Check sheet for the modelled part. Datum: model origin and axes. Units: mm. A direction names the side the tool comes from. Give positions to 0.01 mm unless a question says otherwise; leave off trailing zeros. Loops run counter-clockwise (first coordinate to the right, second up) from the corner with the lowest first, then second, coordinate; pieces in that order, holes last. Notation, with made-up numbers: (-8, 70) -> (8, 70) arc R22 ccw to (8, 94) -> close; hole circle Ø5 at (71, -21.75). An arc over 180 degrees is marked (long way). Answer as CSV lines item,"result". Start each with the question number.
(1) Release check for a two-part mould opening along X. For faces 1 (the face through (3, 6.588, 0)), 2 (the face through (0, 5.588, 0)), 3 (the face through (-0.24, -17.844, 0.462)) record: pulls with the +X half, pulls with the -X half, needs draft (parallel to the pull), parting line crosses it, or undercut.
(2) Gauge pin test, flat ends, axial feed: pin 1 Ø3 at (x, y) = (2, -9) entering from +Z; pin 2 Ø1.5 at (x, y) = (-3, -10.5) entering from +Z; pin 3 Ø2 at (y, z) = (2, 0) entering from +X. Record the tip position at first contact, or that the pin passes through.
(3) Section check A-A on y = -8.75. Enter the section's corners in (x, z), plus the area to 3 significant figures.
(4) Material ranges on line 1 (Z direction, x = 0, y = -6); line 2 (Y direction, x = 5.75, z = -0.75); line 3 (Y direction, x = 0, z = -4.75), recorded low to high. Write a range as from..to.
(5) Access from +Z, -Z, +X, -X, +Y, -Y to the whole of each face (thin tool, end or side, straight path). Record for faces 4 (the face through (-2.86, -7.29, -0.9)), 5 (the face through (-3, 6.588, 0)), 6 (the face through (1, 6, 0)).
from build123d import *

# Parameters (mm, degrees)
CUT_EXTRUDE2_DEPTH = 1


with BuildPart() as part:
    # Sketch2 → Revolve1 (revolve)
    with BuildSketch(Plane.XY, mode=Mode.PRIVATE) as revolve1_sk:
        Polygon((0, -16.412300512), (0, -18.14435132), (3, -16.412300512), (3, 1.587699488), (6.5, 6.587699488), (0, 6.587699488), align=None)
    revolve(revolve1_sk.sketch.rotate(Axis((0, 6.587699488, 0), (0, -1, 0)), 180), axis=Axis((0, 6.587699488, 0), (0, -1, 0)))

    # Sketch4 → Cut-Extrude2 (cut)
    with BuildSketch(Plane(origin=(0, 6.587699488, 0), x_dir=(1, 0, 0), z_dir=(0, 1, 0))):
        Polygon((-1, 6.422616289), (-1, -6.422616289), (-1, -6.622896644), (1, -6.622896644), (1, -6.422616289), (1, 6.422616289), (1, 6.986214166), (-1, 6.986214166), align=None)
    extrude(amount=-CUT_EXTRUDE2_DEPTH, mode=Mode.SUBTRACT)


solid = part.part
Working result:
1,face 1,"needs draft"
1,face 2,"undercut"
1,face 3,"parting line crosses it"
2,pin 1,"stops at z = 2.96"
2,pin 2,"stops at z = 1.98"
2,pin 3,"stops at x = 3.99"
3,outline,"circle Ø6 at (0, 0)"
3,area,"28.3 mm^2"
4,line 1,"z = -3..3"
4,line 2,"y = 5.59..6.59"
4,line 3,"y = 4.09..5.59"
5,face 4,"-Y"
5,face 5,"+Z, -Z, +X, -X, +Y"
5,face 6,"+Z, -Z, +Y"
